Design review of the part built by this model. Coordinates are the model's own, in mm. A direction names the side the tool comes from. Round coordinates to 2 decimals unless told otherwise and drop trailing zeros. Order: outer loops, then holes, each group sorted by start corner. A loop starts at its lowest first (then second) coordinate and runs counter-clockwise, first axis right, second up. Notation, with made-up numbers: (71.25, 9.5) - (129.25, 9.5) arc R16 cw to (129.25, 35.5) - close; hole circle Ø2 at (-34.5, 62.5). An arc over 180 degrees is marked (long way). Use CSV: the item, a comma, the result in double quotes.
from build123d import *

# Parameters (mm, degrees)
F0_W         = 25
F0_H         = 20
F0_W_2       = 15
F0_H_2       = 6.3
F1_DEPTH     = 25
F2_W         = 15
F2_H         = 6.3
F3_DEPTH     = 2
F4_SIZE      = 4
F5_SIZE      = 3
F6_T1_DEPTH  = 15
F6_T6_DEPTH  = 6.1776695297
F6_T11_DEPTH = 6.1776695297


# Not quite as in the source:
# - a fillet or chamfer that OpenCascade refuses, or shapes differently, is made with other operations: its cross-section is extruded or revolved along the edge and cut away or added


with BuildPart() as f1:
    # F0 (on Top) → F1 (new body)
    with BuildSketch(Plane.XY):
        Rectangle(F0_W, F0_H)
        Rectangle(F0_W_2, F0_H_2, mode=Mode.SUBTRACT)
    extrude(amount=F1_DEPTH)

    # F2 (on face) → F3 (join)
    with BuildSketch(Plane(origin=(0, 0, 0), x_dir=(1, 0, 0), z_dir=(0, 0, -1))):
        Rectangle(F2_W, F2_H)
    extrude(amount=-F3_DEPTH)

    # F4
    f4_edges = [f1.edges().sort_by_distance(p)[0] for p in [
        (-7.5, 0, 25),
        (7.5, 0, 25),
        (-12.5, -10, 12.5),
        (12.5, -10, 12.5),
        (12.5, 10, 12.5),
        (-12.5, 10, 12.5),
    ]]
    chamfer(f4_edges, length=F4_SIZE)

    # F5
    f5_edges = [f1.edges().sort_by_distance(p)[0] for p in [
        (0, -3.15, 25),
    ]]
    chamfer(f5_edges, length=F5_SIZE)

    # F6: fillet of radius 5 on 1 edges, made by hand

    # F6_s2 → F6_t1 (cut)
    with BuildSketch(Plane.YZ.offset(-7.5)):
        with BuildLine():
            ThreePointArc((-4.6144660941, 23.4644660941), (-3.5306023374, 21.84234935), (-3.15, 19.9289321881))
            Line((-3.15, 19.9289321881), (-3.15, 22))
            Line((-3.15, 22), (-4.6144660941, 23.4644660941))
        make_face()
    extrude(amount=F6_T1_DEPTH, mode=Mode.SUBTRACT)


with BuildPart() as f6_tool4:
    # F6_s5 → F6_t6 (new body)
    with BuildSketch(Plane.YZ.offset(13.6776695297)):
        with BuildLine():
            ThreePointArc((-4.6144660941, 23.4644660941), (-3.5306023374, 21.84234935), (-3.15, 19.9289321881))
            Line((-3.15, 19.9289321881), (-3.15, 22))
            Line((-3.15, 22), (-4.6144660941, 23.4644660941))
        make_face()
    extrude(amount=-F6_T6_DEPTH)

    split(bisect_by=Plane(origin=(-6.75, 0, 6.75), x_dir=(0, 1, 0), z_dir=(-0.7071067812, 0, 0.7071067812)), keep=Keep.TOP)


with BuildPart() as f1_1:
    add(f1.part)

    # F6_t3: cut F6_tool4
    add(f6_tool4.part, mode=Mode.SUBTRACT)


with BuildPart() as f6_tool9:
    # F6_s10 → F6_t11 (new body)
    with BuildSketch(Plane.YZ.offset(-7.5)):
        with BuildLine():
            ThreePointArc((-4.6144660941, 23.4644660941), (-3.5306023374, 21.84234935), (-3.15, 19.9289321881))
            Line((-3.15, 19.9289321881), (-3.15, 22))
            Line((-3.15, 22), (-4.6144660941, 23.4644660941))
        make_face()
    extrude(amount=-F6_T11_DEPTH)

    split(bisect_by=Plane(origin=(6.75, 0, 6.75), x_dir=(0, 1, 0), z_dir=(0.7071067812, 0, 0.7071067812)), keep=Keep.TOP)


with BuildPart() as f1_2:
    add(f1_1.part)

    # F6_t8: cut F6_tool9
    add(f6_tool9.part, mode=Mode.SUBTRACT)


solid = f1_2.part
1) We need section B-B (y = -2.5). Give the boundary of the cut face in (x, z).
Data:
outline,"(-12.5, 0) - (12.5, 0) - (12.5, 25) - (11.5, 25) - (7.5, 21) - (7.5, 2) - (-7.5, 2) - (-7.5, 21) - (-11.5, 25) - (-12.5, 25) - close"
2) For faces 5 (the face through (0.14, -3.54, 21.87)), 6 (the face through (0, 5, 25)), list the 3-axis set-ups (+Z, -Z, +X, -X, +Y, -Y) from which the entire face can be reached by the end or side of a thin tool; tool diameter is ignored.
Data:
face 5,"+Z"
face 6,"+Z, +X, -X, +Y, -Y"
3) We need section C-C (x = 5). Give the boundary of the cut face in (y, z), then the cut area to 3 significant figures.
Data:
outline,"(-10, 0) - (10, 0) - (10, 25) - (3.15, 25) - (3.15, 2) - (-3.15, 2) - (-3.15, 19.93) arc R5 ccw to (-4.61, 23.46) - (-6.15, 25) - (-10, 25) - close"
area,"350 mm2"
4) The part is to be moulded in two halves that separate along X. For faces 1 (the face through (9.5, -0.5, 23)), 2 (the face through (0, 0, 2)), 3 (the face through (0, 10, 12)), 4 (the face through (12.5, 0, 12)), say which applies: +X half, -X half, draft (parallel to the pull), parting line (faces both ways), or undercut.
Data:
face 1,"undercut"
face 2,"undercut"
face 3,"draft"
face 4,"+X half"
5) To check wall thickness, follow L1, parallel to X at y = -0.5, z = 2.75; L2, parallel to Y at x = -0.5, z = 6; L3, parallel to X at y = -8.5, z = 2.25. State the ranges of each line that lie inside material, in increasing order. Write a range as from..to.
Data:
L1,"x = -12.5..-7.5, 7.5..12.5"
L2,"y = -10..-3.15, 3.15..10"
L3,"x = -10..10"
6) We need section A-A (z = 3.5). Give the boundary of the cut face in (x, y), then the cut area to 4 significant figures.
Data:
outline,"(-12.5, -6) - (-8.5, -10) - (8.5, -10) - (12.5, -6) - (12.5, 6) - (8.5, 10) - (-8.5, 10) - (-12.5, 6) - close; hole (-7.5, -3.15) - (7.5, -3.15) - (7.5, 3.15) - (-7.5, 3.15) - close"
area,"373.5 mm2"
7) Insertion check: pin 1 Ø3 at (x, y) = (-2, -1) entering from +Z. The pin has a flat end and moves straight along its axis. Give the tip position at first contact, or say it passes through.
Data:
pin 1,"stops at z = 2"
8) We need section D-D (z = 21.75). Give the boundary of the cut face in (x, y), then the cut area to 3 significant figures.
Data:
outline,"(-12.5, -6) - (-8.5, -10) - (8.5, -10) - (12.5, -6) - (12.5, 6) - (8.5, 10) - (-8.5, 10) - (-12.5, 6) - close; hole (-8.25, -3.49) - (8.25, -3.49) - (8.25, 3.15) - (-8.25, 3.15) - close"
area,"358 mm2"
